Autodesk Inventor part; units mm, degrees
ref_plane "YZ Plane" through (0, 0, 0) normal (1, 0, 0) x (0, 1, 0)
ref_plane "XZ Plane" through (0, 0, 0) normal (0, 1, 0) x (-1, 0, 0)
ref_plane "XY Plane" through (0, 0, 0) normal (0, 0, 1) x (1, 0, 0)
sketch "Skizze1" plane through (0, 0, 0) normal (0, 0, 1) x (1, 0, 0)
  line L0 (-24, 0) -> (144, 0)
  line L1 (0, -21) -> (0, 126)
  line L2 (0, 0) -> (120, 0)
  line L3 (120, 0) -> (120, 105)
  line L4 (120, 105) -> (0, 105)
  line L5 (0, 105) -> (0, 0)
  line L6 (10, 10) -> (110, 10)
  line L7 (110, 10) -> (110, 95)
  line L8 (110, 95) -> (10, 95)
  line L9 (10, 95) -> (10, 10)
  dimension "d0" = 85
  dimension "d1" = 100
  dimension "d2" = 10
  dimension "d3" = 10
  dimension "d4" = 10
  dimension "d5" = 10
extrude "Extrusion1" add sketch "Skizze1" along normal blind 160
sketch "Skizze2" plane through (0, 0, 0) normal (0, 0, -1) x (-1, 0, 0)
  line L0 (-120, 0) -> (-120, 105)
  line L1 (-120, 105) -> (0, 105)
  line L2 (-120, 0) -> (0, 0)
  line L3 (0, 0) -> (0, 105)
  line L4 (0, 105) -> (-120, 105)
  line L5 (-120, 105) -> (-120, 0)
  point P0 (0, 0)
extrude "Extrusion2" add sketch "Skizze2" against normal blind 10
sketch "Skizze3" plane through (0, 0, 160) normal (-1, 0, 0) x (0, 0, 1)
  line L0 (-120, 95) -> (-150, 95)
  line L1 (-150, 95) -> (-150, 10)
  line L2 (-150, 10) -> (-120, 10)
  line L3 (-120, 10) -> (-120, 95)
  line L4 (-160, 105) -> (-160, 0)
  line L5 (-160, 0) -> (0, 0)
  line L6 (-160, 105) -> (0, 105)
  dimension "d10" = 10
  dimension "d11" = 10
  dimension "d12" = 10
  dimension "d13" = 30
extrude "Extrusion3" cut sketch "Skizze3" against normal blind 10
sketch "Skizze4" plane through (0, 0, 160) normal (-1, 0, 0) x (0, 0, 1)
  line L0 (-160, 105) -> (0, 105)
  line L1 (-160, 0) -> (0, 0)
  line L2 (-100, 105) -> (-110, 105)
  line L3 (-110, 105) -> (-110, 0)
  line L4 (-110, 0) -> (-100, 0)
  line L5 (-100, 0) -> (-100, 105)
  line L6 (-120, 95) -> (-120, 10)
  dimension "d16" = 10
  dimension "d17" = 10
extrude "Extrusion4" add sketch "Skizze4" against normal blind 120
sketch "Skizze5" plane through (0, 0, 160) normal (0, 0, 1) x (1, 0, 0)
  line L0 (117.6, 102.6) -> (2.4, 102.6)
  line L1 (2.4, 102.6) -> (2.4, 2.4)
  line L2 (2.4, 2.4) -> (117.6, 2.4)
  line L3 (117.6, 2.4) -> (117.6, 102.6)
  line L4 (112.4, 97.4) -> (7.6, 97.4)
  line L5 (7.6, 97.4) -> (7.6, 7.6)
  line L6 (7.6, 7.6) -> (112.4, 7.6)
  line L7 (112.4, 7.6) -> (112.4, 97.4)
  line L8 (120, 0) -> (120, 105)
  line L9 (0, 0) -> (120, 0)
  line L10 (110, 95) -> (110, 10)
  line L11 (110, 10) -> (10, 10)
  line L12 (120, 105) -> (0, 105)
  line L13 (10, 95) -> (110, 95)
  line L14 (10, 10) -> (10, 95)
  line L15 (0, 105) -> (0, 0)
  dimension "d20" = 2.4
  dimension "d21" = 2.4
  dimension "d22" = 2.4
  dimension "d23" = 2.4
  dimension "d24" = 2.4
  dimension "d25" = 2.4
  dimension "d26" = 2.4
  dimension "d27" = 2.4
extrude "Extrusion5" cut sketch "Skizze5" against normal blind 7.5 contours L3 L2 L1 L0
sketch "Skizze6" plane through (0, 0, 160) normal (-1, 0, 0) x (0, 0, 1)
  line L0 (-120, 10) -> (-120, 95)
  line L1 (-150, 95) -> (-150, 10)
  line L2 (-120, 95) -> (-150, 95)
  line L3 (-150, 95) -> (-150, 10)
  line L4 (-150, 10) -> (-120, 10)
  line L5 (-120, 10) -> (-120, 95)
  point P0 (-160, 0)
extrude "Extrusion6" add sketch "Skizze6" against normal blind 10
sketch "Skizze7" plane through (0, 0, 160) normal (0, -1, 0) x (1, 0, 0)
  line L0 (10, -120) -> (110, -120)
  line L1 (110, -120) -> (110, -150)
  line L2 (110, -150) -> (10, -150)
  line L3 (10, -150) -> (10, -120)
  line L4 (0, -160) -> (120, -160)
  line L5 (120, -160) -> (120, 0)
  line L6 (0, -160) -> (0, 0)
  dimension "d32" = 10
  dimension "d33" = 10
  dimension "d34" = 10
  dimension "d35" = 30
extrude "Extrusion7" cut sketch "Skizze7" against normal blind 10
properties part number "Eierkocher_final" material "Acetalharz, Schwarz"
Could you check a few things on this model? Use its own coordinates, in mm. A direction names the side the tool comes from. Give positions to 0.01 mm unless a question says otherwise; leave off trailing zeros. Order: outer loops, then holes, each group sorted by start corner. A loop starts at its lowest first (then second) coordinate and runs counter-clockwise, first axis right, second up. Notation, with made-up numbers: (22.25, 22) - (39.25, 22) arc R29 cw to (39.25, 54) - close; hole circle Ø3 at (4.5, 47.25). An arc over 180 degrees is marked (long way). Return JSON: item names as keys, results as strings. Group by question number.
Q1. Which directions (+Z, -Z, +X, -X, +Y, -Y) give clear straight access to the entire face, cutting with the end or side of a thin tool? Please do faces 1 (the face through (2, 53, 160)), 2 (the face through (110, 52, 109)), 3 (the face through (59, 95, 30)).
Q2. Thinking about a two-plate mould opening in Z: for faces 4 (the face through (59, 53, 0)), 5 (the face through (0, 53, 79)), 6 (the face through (59, 5, 40)), which applies, pulls with the +Z half, pulls with the -Z half, needs draft (parallel to the pull), parting line crosses it, or undercut?
Q3. Suppose I cut it at B-B, the plane y = 63.5. Please give me the cut outline in (x, z).
Q4. Please list where these lines run through material, in increasing order: line 1 along X through (y, z) = (97, 153); line 2 along Z through (x, y) = (70.5, 94); line 3 along Y through (x, z) = (59, 100). Write a range as [from, to].
Q5. Suppose I cut it at D-D, the plane x = 18. Please give me the cut outline in (y, z).
Q6. Suppose I cut it at A-A, the plane z = 69.5. Please give me the cut outline in (x, y).
Q7. Suppose I cut it at C-C, the plane z = 30.5. Please give me the cut outline in (x, y).
Resolved:
{
 "1": {"face 1": "+Z, +X, -X, +Y, -Y", "face 2": "+Z", "face 3": "none"},
 "2": {"face 4": "pulls with the -Z half", "face 5": "needs draft", "face 6": "undercut"},
 "3": {"outline": "(0, 0) - (120, 0) - (120, 160) - (117.6, 160) - (117.6, 152.5) - (112.4, 152.5) - (112.4, 160) - (110, 160) - (110, 60) - (10, 60) - (10, 160) - (7.6, 160) - (7.6, 152.5) - (2.4, 152.5) - (2.4, 160) - (0, 160) - close; hole (10, 10) - (110, 10) - (110, 50) - (10, 50) - close"},
 "4": {"line 1": "x = [0, 2.4], [7.6, 112.4], [117.6, 120]", "line 2": "z = [0, 10], [50, 60]", "line 3": "y = [0, 10], [95, 105]"},
 "5": {"outline": "(0, 0) - (105, 0) - (105, 160) - (102.6, 160) - (102.6, 152.5) - (97.4, 152.5) - (97.4, 160) - (95, 160) - (95, 60) - (10, 60) - (10, 160) - (7.6, 160) - (7.6, 152.5) - (2.4, 152.5) - (2.4, 160) - (0, 160) - (0, 40) - (10, 40) - (10, 50) - (95, 50) - (95, 10) - (0, 10) - close"},
 "6": {"outline": "(0, 0) - (120, 0) - (120, 105) - (0, 105) - close; hole (10, 10) - (110, 10) - (110, 95) - (10, 95) - close"},
 "7": {"outline": "(0, 0) - (10, 0) - (10, 95) - (110, 95) - (110, 0) - (120, 0) - (120, 105) - (0, 105) - close"}
}
